```python
from build123d import *

# Parameters (mm, degrees)
SKETCH1_R           = 5
BOSS_EXTRUDE1_DEPTH = 12.7


with BuildPart() as part:
    # Sketch1 → Boss-Extrude1 (new body)
    with BuildSketch(Plane.XY):
        Polygon((-38.1, -34.544), (-15.875, -34.544), (-15.875, -21.844), (0, -21.844), (15.875, -21.844), (15.875, -34.544), (38.1, -34.544), (38.1, 28.336368082), (-19.05, 28.336368082), (-38.1, 28.336368082), align=None)
        with BuildLine():
            ThreePointArc((8.5, -8.264), (6.01040764, -14.27440764), (0, -16.764))
            ThreePointArc((0, -16.764), (-6.01040764, -2.25359236), (8.5, -8.264))
        make_face(mode=Mode.SUBTRACT)
        with Locations((-19.05, 7.992)):
            Circle(SKETCH1_R, mode=Mode.SUBTRACT)
        with Locations((19.05, 7.992)):
            Circle(SKETCH1_R, mode=Mode.SUBTRACT)
    extrude(amount=BOSS_EXTRUDE1_DEPTH)


solid = part.part
```
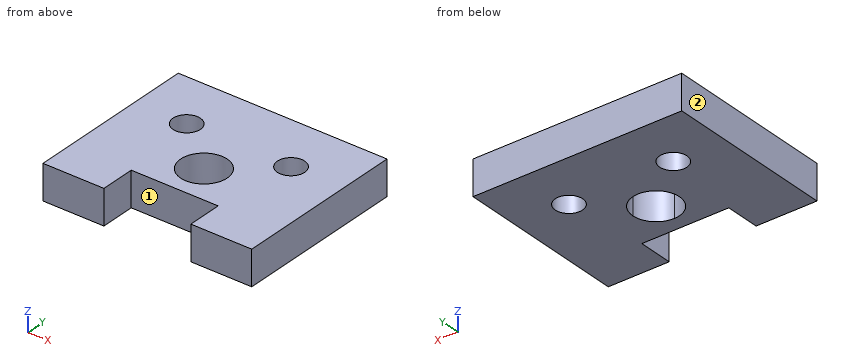
Here's how the part is built. I have some questions about the finished solid (model axes, mm). Face numbers are marked on the shaded views. A direction names the side the tool comes from. Coordinates: 2 decimals unless noted, no trailing zeros. Order: outer loops, then holes, each group sorted by start corner. A loop starts at its lowest first (then second) coordinate and runs counter-clockwise, first axis right, second up.
1) Imagine slicing it at A-A on x = 19.05. List the corners of the cut face in (y, z) for me, and give its area (3 significant figures).
2) I need wall thicknesses on line 1 (Y direction, x = 0, z = 3); line 2 (Y direction, x = 19.05, z = 2.75); line 3 (X direction, y = 11, z = 4.25). Which ranges of each line are inside material? Lowest first, please.
3) Which directions (+Z, -Z, +X, -X, +Y, -Y) give clear straight access to the entire face, cutting with the end or side of a thin tool? Please do the marked faces 1 and 2.
4) Imagine slicing it at C-C on z = 8.5. List the corners of the cut face in (x, y) for me (3 decimals), and give its area (3 significant figures).
5) Imagine slicing it at B-B on y = -15. List the corners of the cut face in (x, z) for me, and give its area (3 significant figures).
6) Will this pin go through, and if not, where does the flat tip stop? pin 1 (6.5 mm diameter, centred on x = 1.5, z = 4.5, fed in from -Y).
Response values:
1. outline: (-34.54, 0) - (2.99, 0) - (2.99, 12.7) - (-34.54, 12.7) - close; (12.99, 0) - (28.34, 0) - (28.34, 12.7) - (12.99, 12.7) - close
1. area: 672 mm2
2. line 1: y = -21.84 to -16.76, 0.24 to 28.34
2. line 2: y = -34.54 to 2.99, 12.99 to 28.34
2. line 3: x = -38.1 to -23.04, -15.06 to 15.06, 23.04 to 38.1
3. face 1: +Z, -Z, -Y
3. face 2: +Z, -Z, -X, +Y, -Y
4. outline: (-38.1, -34.544) - (-15.875, -34.544) - (-15.875, -21.844) - (15.875, -21.844) - (15.875, -34.544) - (38.1, -34.544) - (38.1, 28.336) - (-38.1, 28.336) - close; hole circle Ø10 at (-19.05, 7.992); hole circle Ø17 at (0, -8.264); hole circle Ø10 at (19.05, 7.992)
4. area: 4,000 mm2
5. outline: (-38.1, 0) - (-5.18, 0) - (-5.18, 12.7) - (-38.1, 12.7) - close; (5.18, 0) - (38.1, 0) - (38.1, 12.7) - (5.18, 12.7) - close
5. area: 836 mm2
6. pin 1: stops at y = -21.84
